Design review of the part built by this model. Coordinates are the model's own, in mm. Face numbers are marked on the shaded views. Coordinates: 2 decimals unless noted, no trailing zeros. Loops run counter-clockwise (first coordinate to the right, second up) from the corner with the lowest first, then second, coordinate; pieces in that order, holes last. Notation, with made-up numbers: M 2.5,26.25 L 30.5,26.25 A3 cw 30.5,30.25 Z; hole C -14,58 d7. An arc over 180 degrees is marked long. Put each result on its own line as item: value. Start each with the question number.
(1) Take a section at B-B, the plane y = 0. Give the boundary of the cut face in (x, z), then the cut area to 3 significant figures.
(2) The part is to be moulded in two halves that separate along Y. For the marked faces 1 and 2, say which applies: +Y half, -Y half, draft (parallel to the pull), parting line (faces both ways), or undercut.
(3) Take a section at A-A, the plane x = -1.75. Give the boundary of the cut face in (y, z), then the cut area to 3 significant figures.
(4) Clearance check with flat-ended pins moving along their axes: pin 1 (1 mm diameter, centred on x = -8, z = 75, fed in from -Y); pin 2 (5 mm diameter, centred on x = 7, y = -1, fed in from +Z); pin 3 (5 mm diameter, centred on x = -7.5, y = -3, fed in from -Z). State where each tip first meets the part, or that it passes through.
(5) Take a section at D-D, the plane y = 8.75. Give the boundary of the cut face in (x, z).
(6) For probe 1 along X at (y, z) = (0, 63.5); probe 2 along Z at (x, y) = (3, -6.5), list the stretches that pass through material, from the lowest coordinate up. Write a range as [from, to].
(7) Take a section at C-C, the plane z = 84.5. Give the boundary of the cut face in (x, y), then the cut area to 3 significant figures.
Autodesk Inventor part; units mm, degrees
ref_plane "Start Plane" through (0, 0, -8.6396) normal (0, 0, 1) x (1, 0, 0)
ref_plane "End Plane" through (0, 0, 120.1752) normal (0, 0, 1) x (1, 0, 0)
ref_plane "Work Plane4" through (6.5224, -8.4419, 117.6947) normal (-0.3057, 0.3957, 0.866) x (0.9499, 0.0648, 0.3057)
ref_plane "Start Plane" through (0, 0, -8.6396) normal (0, 0, 1) x (1, 0, 0)
ref_plane "End Plane" through (0, 0, 120.1752) normal (0, 0, 1) x (1, 0, 0)
sketch "Sketch" plane through (0, 0, 0) normal (0, 0, 1) x (1, 0, 0)
  circle A0 centre (0, 0) radius 6.9342
  circle A1 centre (0, 0) radius 10.668
  dimension "d0" = 21.336
  dimension "d1" = 3.7338
extrude "Body" add sketch "Sketch" along normal up to surface (128.8148 mm away) from surface at -8.6396
sketch "Sketch3" plane through (0, 0, 0) normal (0, 0, 1) x (1, 0, 0)
  line L0 (0, 0) -> (10, 0)
ref_plane "Work Plane3" through (0, 0, 0) normal (0, -1, 0) x (1, 0, 0)
sketch "Sketch4" plane through (0, 0, 0) normal (0, -1, 0) x (1, 0, 0)
  line L0 (-2, -8.6396) -> (12, -8.6396)
  line L1 (-2, 120.1752) -> (12, 120.1752)
  dimension "d7" = 128.8148
ref_plane "Work Plane4" through (6.5224, -8.4419, 117.6947) normal (-0.3057, 0.3957, 0.866) x (0.9499, 0.0648, 0.3057)
split "Split1" plane through (6.5224, -8.4419, 117.6947) removes the side toward (-0.3057, 0.3957, 0.866)
ref_plane "Work Plane5" through (6.5224, -8.4419, -6.1592) normal (-0.3057, 0.3957, -0.866) x (0.3025, 0.9028, 0.3057)
split "Split2" plane through (6.5224, -8.4419, -6.1592) removes the side toward (-0.3057, 0.3957, -0.866)
equation "\"d0\" = G_H"
equation "\"d1\" = G_T"
equation "\"d2\" = G_L"
equation "\"G_H\" = 21.336"
equation "\"G_T\" = 3.7338"
equation "\"G_L\" = 123.85392"
equation "\"G_OFFSET_START\" = 8.6396"
equation "\"G_OFFSET_END\" = 8.6396"
equation "\"d4\" = -G_OFFSET_START"
equation "\"d5\" = G_OFFSET_END + B_L"
equation "\"B_L\" = 111.53557"
properties part number "ANSI - 1/2 x 0.147 - 4.876" material "Steel, Mild"
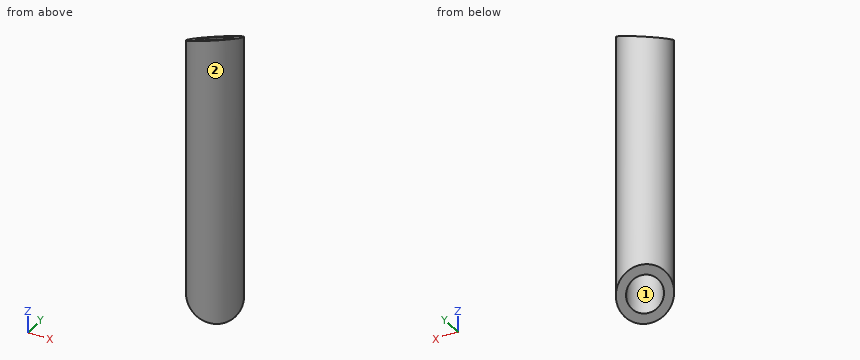
Computed values:
1. outline: M -10.67,3.77 L -6.93,2.45 L -6.93,109.09 L -10.67,107.77 Z; M 6.93,-2.45 L 10.67,-3.77 L 10.67,115.3 L 6.93,113.98 Z
1. area: 833 mm^2
2. face 1: undercut
2. face 2: parting line
3. outline: M -10.52,-4.19 L -6.71,-2.45 L -6.71,113.98 L -10.52,115.73 Z; M 6.71,3.68 L 10.52,5.43 L 10.52,106.11 L 6.71,107.85 Z
3. area: 841 mm^2
4. pin 1: stops at y = -7.59
4. pin 2: stops at z = 115.91
4. pin 3: stops at z = -0.17
5. outline: M -6.1,6.15 L 6.1,1.84 L 6.1,109.69 L -6.1,105.38 Z
6. probe 1: x = [-10.67, -6.93], [6.93, 10.67]
6. probe 2: z = [-4.03, 115.56]
7. outline: C 0,0 d21.34; hole C 0,0 d13.87
7. area: 206 mm^2
